Could you check a few things on this drawing? It's one solid part, dimensions in mm from its lowest x, y, z. A direction names the side the tool comes from. Round coordinates to 2 decimals unless told otherwise and drop trailing zeros. Write each loop counter-clockwise with the first axis right and the second up, starting at its lowest first coordinate (ties: lowest second). Pieces come first, ordered by that corner, then holes. Notation, with made-up numbers: (12.5, 8) -> (58.5, 8) arc R20 cw to (58.5, 40) -> close; hole circle Ø9 at (-4, 79). An arc over 180 degrees is marked (long way). Return JSON: item names as keys, results as strings.
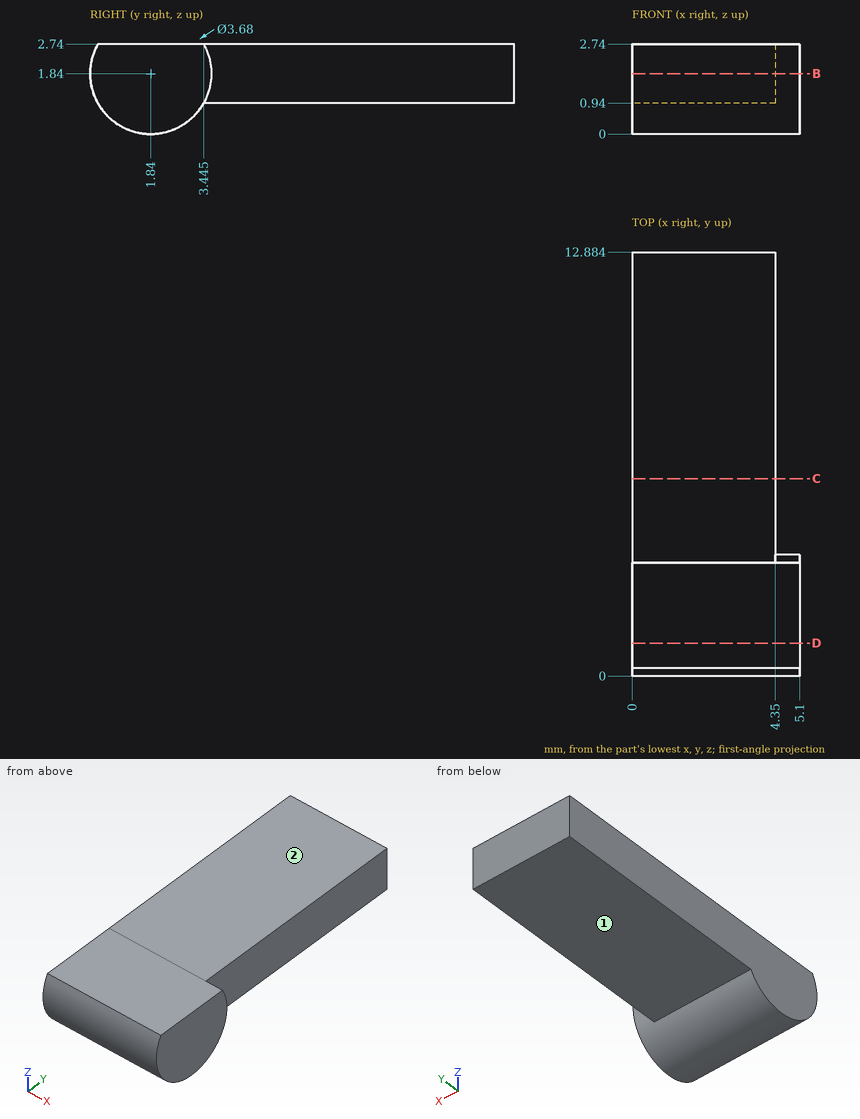
1) Will these pins go through, and if not, where does the flat tip stop? pin 1 Ø2 at (x, y) = (3, 3) entering from -Z; pin 2 Ø1.4 at (y, z) = (9.5, 1.5) entering from +X.
Return value:
{"pin 1": "z = 0.01", "pin 2": "x = 4.35"}
2) I want a section at D-D, the plane y = 1. Please give me the cut outline in (x, z).
Return value:
{"outline": "(0, 0.2) -> (5.1, 0.2) -> (5.1, 2.74) -> (0, 2.74) -> close"}
3) I want a section at C-C, the plane y = 6. Please give me the cut outline in (x, z).
Return value:
{"outline": "(0, 0.94) -> (4.35, 0.94) -> (4.35, 2.74) -> (0, 2.74) -> close"}
4) I want a section at B-B, the plane z = 1.84. Please give me the cut outline in (x, y), and give its area (3 significant figures).
Return value:
{"outline": "(0, 0) -> (5.1, 0) -> (5.1, 3.68) -> (4.35, 3.68) -> (4.35, 12.88) -> (0, 12.88) -> close", "area": "58.8 mm²"}
5) If I drill on probe 1 along X at (y, z) = (5.25, 1.25); probe 2 along Z at (x, y) = (1.25, 4.25); probe 3 along Y at (x, z) = (3.1, 2.6) (1 decimal), over which ranges is the centre line in solid material (lowest first)? Write a range as [from, to].
Return value:
{"probe 1": "[0, 4.35]", "probe 2": "[0.94, 2.74]", "probe 3": "[0.2, 12.9]"}
6) For the marked faces 1 and 2, which set-ups out of +Z, -Z, +X, -X, +Y, -Y let a thin tool reach every point of the face, with its end or its side?
Return value:
{"face 1": "-Z, +X, -X, +Y", "face 2": "+Z, +X, -X, +Y, -Y"}
